```python
from build123d import *
from OCP.BRepFilletAPI import BRepFilletAPI_MakeChamfer

# Parameters (mm, degrees)
SKETCH1_W                   = 2.54
SKETCH1_H                   = 2.5
BOSS_EXTRUDE1_DEPTH         = 8.5
SKETCH2_W                   = 2.54
SKETCH2_H                   = 1.2
CUT_EXTRUDE1_DEPTH          = 0.3
CUT_EXTRUDE2_START          = -6
SKETCH3_W                   = 0.64
SKETCH3_H                   = 0.64
CUT_EXTRUDE2_DEPTH          = 15.68477979
CHAMFER1_SIZE               = 0.5
SKETCH4_W                   = 0.64
SKETCH4_H                   = 0.4
BOSS_EXTRUDE2_DEPTH         = 3.8
CHAMFER2_SIZE               = 1
CHAMFER2_SIZE2              = 0.15838444
LPATTERN1_COUNT             = 9
LPATTERN1_PITCH             = 2.54
CHAMFER1_OF_LPATTERN1_SIZE  = 0.5
CHAMFER2_OF_LPATTERN1_SIZE  = 1
CHAMFER2_OF_LPATTERN1_SIZE2 = 0.15838444


with BuildPart() as part:
    # Sketch1 → Boss-Extrude1 (new body)
    with BuildSketch(Plane(origin=(0, 0, 0), x_dir=(1, 0, 0), z_dir=(0, 1, 0))):
        Rectangle(SKETCH1_W, SKETCH1_H)
    boss_extrude1 = extrude(amount=BOSS_EXTRUDE1_DEPTH)

    # Sketch2 → Cut-Extrude1 (cut)
    with BuildSketch(Plane.XZ):
        Rectangle(SKETCH2_W, SKETCH2_H)
    cut_extrude1 = extrude(amount=-CUT_EXTRUDE1_DEPTH, mode=Mode.SUBTRACT)

    # Sketch3 → Cut-Extrude2 (cut)
    with BuildSketch(Plane(origin=(0, 8.5, 0), x_dir=(1, 0, 0), z_dir=(0, 1, 0)).offset(CUT_EXTRUDE2_START)):
        Rectangle(SKETCH3_W, SKETCH3_H)
    cut_extrude2 = extrude(amount=CUT_EXTRUDE2_DEPTH, mode=Mode.SUBTRACT)

    # Chamfer1
    chamfer1_edges = [part.edges().sort_by_distance(p)[0] for p in [
        (0, 8.5, 0.32),
        (-0.32, 8.5, 0),
        (0, 8.5, -0.32),
        (0.32, 8.5, 0),
    ]]
    chamfer(chamfer1_edges, length=CHAMFER1_SIZE)

    # Sketch4 → Boss-Extrude2 (add)
    with BuildSketch(Plane.XZ.offset(-0.3)):
        Rectangle(SKETCH4_W, SKETCH4_H)
    boss_extrude2 = extrude(amount=BOSS_EXTRUDE2_DEPTH)

    # Chamfer2: one chamfer whose edges measure the first distance from different faces: ONE call of the kernel's chamfer builder (chamfer() names one face for all edges)
    chamfer2_edges_1 = [part.edges().sort_by_distance(p)[0] for p in [
        (0.32, -3.5, 0),
    ]]
    chamfer2_side_1 = [part.faces().sort_by_distance(p)[0] for p in [
        (0.32, -1.6, 0),
    ]]
    chamfer2_edges_2 = [part.edges().sort_by_distance(p)[0] for p in [
        (-0.32, -3.5, 0),
    ]]
    chamfer2_side_2 = [part.faces().sort_by_distance(p)[0] for p in [
        (-0.32, -1.6, 0),
    ]]
    chamfer2 = BRepFilletAPI_MakeChamfer(part.part.solid().wrapped)
    for e in chamfer2_edges_1:
        chamfer2.Add(CHAMFER2_SIZE, CHAMFER2_SIZE2, e.wrapped, chamfer2_side_1[0].wrapped)  # the first distance lies on this face
    for e in chamfer2_edges_2:
        chamfer2.Add(CHAMFER2_SIZE, CHAMFER2_SIZE2, e.wrapped, chamfer2_side_2[0].wrapped)  # the first distance lies on this face
    add(Compound.cast(chamfer2.Shape()), mode=Mode.REPLACE)

    # LPattern1: Boss-Extrude1, Cut-Extrude1, Cut-Extrude2, Boss-Extrude2 ×9
    with Locations(*[(-i * LPATTERN1_PITCH, 0, 0) for i in range(1, LPATTERN1_COUNT)]):
        add(boss_extrude1)
        add(cut_extrude1, mode=Mode.SUBTRACT)
        add(cut_extrude2, mode=Mode.SUBTRACT)
        add(boss_extrude2)

    # Chamfer1 of LPattern1
    chamfer1_of_lpattern1_edges = [part.edges().sort_by_distance(p)[0] for p in [
        (-2.54, 8.5, 0.32),
        (-2.86, 8.5, 0),
        (-2.54, 8.5, -0.32),
        (-2.22, 8.5, 0),
        (-5.08, 8.5, 0.32),
        (-5.4, 8.5, 0),
        (-5.08, 8.5, -0.32),
        (-4.76, 8.5, 0),
        (-7.62, 8.5, 0.32),
        (-7.94, 8.5, 0),
        (-7.62, 8.5, -0.32),
        (-7.3, 8.5, 0),
        (-10.16, 8.5, 0.32),
        (-10.48, 8.5, 0),
        (-10.16, 8.5, -0.32),
        (-9.84, 8.5, 0),
        (-12.7, 8.5, 0.32),
        (-13.02, 8.5, 0),
        (-12.7, 8.5, -0.32),
        (-12.38, 8.5, 0),
        (-15.24, 8.5, 0.32),
        (-15.56, 8.5, 0),
        (-15.24, 8.5, -0.32),
        (-14.92, 8.5, 0),
        (-17.78, 8.5, 0.32),
        (-18.1, 8.5, 0),
        (-17.78, 8.5, -0.32),
        (-17.46, 8.5, 0),
        (-20.32, 8.5, 0.32),
        (-20.64, 8.5, 0),
        (-20.32, 8.5, -0.32),
        (-20, 8.5, 0),
    ]]
    chamfer(chamfer1_of_lpattern1_edges, length=CHAMFER1_OF_LPATTERN1_SIZE)

    # Chamfer2 of LPattern1: one chamfer whose edges measure the first distance from different faces: ONE call of the kernel's chamfer builder (chamfer() names one face for all edges)
    chamfer2_of_lpattern1_edges_1 = [part.edges().sort_by_distance(p)[0] for p in [
        (-2.22, -3.5, 0),
    ]]
    chamfer2_of_lpattern1_side_1 = [part.faces().sort_by_distance(p)[0] for p in [
        (-2.22, -1.6, 0),
    ]]
    chamfer2_of_lpattern1_edges_2 = [part.edges().sort_by_distance(p)[0] for p in [
        (-2.86, -3.5, 0),
    ]]
    chamfer2_of_lpattern1_side_2 = [part.faces().sort_by_distance(p)[0] for p in [
        (-2.86, -1.6, 0),
    ]]
    chamfer2_of_lpattern1_edges_3 = [part.edges().sort_by_distance(p)[0] for p in [
        (-4.76, -3.5, 0),
    ]]
    chamfer2_of_lpattern1_side_3 = [part.faces().sort_by_distance(p)[0] for p in [
        (-4.76, -1.6, 0),
    ]]
    chamfer2_of_lpattern1_edges_4 = [part.edges().sort_by_distance(p)[0] for p in [
        (-5.4, -3.5, 0),
    ]]
    chamfer2_of_lpattern1_side_4 = [part.faces().sort_by_distance(p)[0] for p in [
        (-5.4, -1.6, 0),
    ]]
    chamfer2_of_lpattern1_edges_5 = [part.edges().sort_by_distance(p)[0] for p in [
        (-7.3, -3.5, 0),
    ]]
    chamfer2_of_lpattern1_side_5 = [part.faces().sort_by_distance(p)[0] for p in [
        (-7.3, -1.6, 0),
    ]]
    chamfer2_of_lpattern1_edges_6 = [part.edges().sort_by_distance(p)[0] for p in [
        (-7.94, -3.5, 0),
    ]]
    chamfer2_of_lpattern1_side_6 = [part.faces().sort_by_distance(p)[0] for p in [
        (-7.94, -1.6, 0),
    ]]
    chamfer2_of_lpattern1_edges_7 = [part.edges().sort_by_distance(p)[0] for p in [
        (-9.84, -3.5, 0),
    ]]
    chamfer2_of_lpattern1_side_7 = [part.faces().sort_by_distance(p)[0] for p in [
        (-9.84, -1.6, 0),
    ]]
    chamfer2_of_lpattern1_edges_8 = [part.edges().sort_by_distance(p)[0] for p in [
        (-10.48, -3.5, 0),
    ]]
    chamfer2_of_lpattern1_side_8 = [part.faces().sort_by_distance(p)[0] for p in [
        (-10.48, -1.6, 0),
    ]]
    chamfer2_of_lpattern1_edges_9 = [part.edges().sort_by_distance(p)[0] for p in [
        (-12.38, -3.5, 0),
    ]]
    chamfer2_of_lpattern1_side_9 = [part.faces().sort_by_distance(p)[0] for p in [
        (-12.38, -1.6, 0),
    ]]
    chamfer2_of_lpattern1_edges_10 = [part.edges().sort_by_distance(p)[0] for p in [
        (-13.02, -3.5, 0),
    ]]
    chamfer2_of_lpattern1_side_10 = [part.faces().sort_by_distance(p)[0] for p in [
        (-13.02, -1.6, 0),
    ]]
    chamfer2_of_lpattern1_edges_11 = [part.edges().sort_by_distance(p)[0] for p in [
        (-14.92, -3.5, 0),
    ]]
    chamfer2_of_lpattern1_side_11 = [part.faces().sort_by_distance(p)[0] for p in [
        (-14.92, -1.6, 0),
    ]]
    chamfer2_of_lpattern1_edges_12 = [part.edges().sort_by_distance(p)[0] for p in [
        (-15.56, -3.5, 0),
    ]]
    chamfer2_of_lpattern1_side_12 = [part.faces().sort_by_distance(p)[0] for p in [
        (-15.56, -1.6, 0),
    ]]
    chamfer2_of_lpattern1_edges_13 = [part.edges().sort_by_distance(p)[0] for p in [
        (-17.46, -3.5, 0),
    ]]
    chamfer2_of_lpattern1_side_13 = [part.faces().sort_by_distance(p)[0] for p in [
        (-17.46, -1.6, 0),
    ]]
    chamfer2_of_lpattern1_edges_14 = [part.edges().sort_by_distance(p)[0] for p in [
        (-18.1, -3.5, 0),
    ]]
    chamfer2_of_lpattern1_side_14 = [part.faces().sort_by_distance(p)[0] for p in [
        (-18.1, -1.6, 0),
    ]]
    chamfer2_of_lpattern1_edges_15 = [part.edges().sort_by_distance(p)[0] for p in [
        (-20, -3.5, 0),
    ]]
    chamfer2_of_lpattern1_side_15 = [part.faces().sort_by_distance(p)[0] for p in [
        (-20, -1.6, 0),
    ]]
    chamfer2_of_lpattern1_edges_16 = [part.edges().sort_by_distance(p)[0] for p in [
        (-20.64, -3.5, 0),
    ]]
    chamfer2_of_lpattern1_side_16 = [part.faces().sort_by_distance(p)[0] for p in [
        (-20.64, -1.6, 0),
    ]]
    chamfer2_of_lpattern1 = BRepFilletAPI_MakeChamfer(part.part.solid().wrapped)
    for e in chamfer2_of_lpattern1_edges_1:
        chamfer2_of_lpattern1.Add(CHAMFER2_OF_LPATTERN1_SIZE, CHAMFER2_OF_LPATTERN1_SIZE2, e.wrapped, chamfer2_of_lpattern1_side_1[0].wrapped)  # the first distance lies on this face
    for e in chamfer2_of_lpattern1_edges_2:
        chamfer2_of_lpattern1.Add(CHAMFER2_OF_LPATTERN1_SIZE, CHAMFER2_OF_LPATTERN1_SIZE2, e.wrapped, chamfer2_of_lpattern1_side_2[0].wrapped)  # the first distance lies on this face
    for e in chamfer2_of_lpattern1_edges_3:
        chamfer2_of_lpattern1.Add(CHAMFER2_OF_LPATTERN1_SIZE, CHAMFER2_OF_LPATTERN1_SIZE2, e.wrapped, chamfer2_of_lpattern1_side_3[0].wrapped)  # the first distance lies on this face
    for e in chamfer2_of_lpattern1_edges_4:
        chamfer2_of_lpattern1.Add(CHAMFER2_OF_LPATTERN1_SIZE, CHAMFER2_OF_LPATTERN1_SIZE2, e.wrapped, chamfer2_of_lpattern1_side_4[0].wrapped)  # the first distance lies on this face
    for e in chamfer2_of_lpattern1_edges_5:
        chamfer2_of_lpattern1.Add(CHAMFER2_OF_LPATTERN1_SIZE, CHAMFER2_OF_LPATTERN1_SIZE2, e.wrapped, chamfer2_of_lpattern1_side_5[0].wrapped)  # the first distance lies on this face
    for e in chamfer2_of_lpattern1_edges_6:
        chamfer2_of_lpattern1.Add(CHAMFER2_OF_LPATTERN1_SIZE, CHAMFER2_OF_LPATTERN1_SIZE2, e.wrapped, chamfer2_of_lpattern1_side_6[0].wrapped)  # the first distance lies on this face
    for e in chamfer2_of_lpattern1_edges_7:
        chamfer2_of_lpattern1.Add(CHAMFER2_OF_LPATTERN1_SIZE, CHAMFER2_OF_LPATTERN1_SIZE2, e.wrapped, chamfer2_of_lpattern1_side_7[0].wrapped)  # the first distance lies on this face
    for e in chamfer2_of_lpattern1_edges_8:
        chamfer2_of_lpattern1.Add(CHAMFER2_OF_LPATTERN1_SIZE, CHAMFER2_OF_LPATTERN1_SIZE2, e.wrapped, chamfer2_of_lpattern1_side_8[0].wrapped)  # the first distance lies on this face
    for e in chamfer2_of_lpattern1_edges_9:
        chamfer2_of_lpattern1.Add(CHAMFER2_OF_LPATTERN1_SIZE, CHAMFER2_OF_LPATTERN1_SIZE2, e.wrapped, chamfer2_of_lpattern1_side_9[0].wrapped)  # the first distance lies on this face
    for e in chamfer2_of_lpattern1_edges_10:
        chamfer2_of_lpattern1.Add(CHAMFER2_OF_LPATTERN1_SIZE, CHAMFER2_OF_LPATTERN1_SIZE2, e.wrapped, chamfer2_of_lpattern1_side_10[0].wrapped)  # the first distance lies on this face
    for e in chamfer2_of_lpattern1_edges_11:
        chamfer2_of_lpattern1.Add(CHAMFER2_OF_LPATTERN1_SIZE, CHAMFER2_OF_LPATTERN1_SIZE2, e.wrapped, chamfer2_of_lpattern1_side_11[0].wrapped)  # the first distance lies on this face
    for e in chamfer2_of_lpattern1_edges_12:
        chamfer2_of_lpattern1.Add(CHAMFER2_OF_LPATTERN1_SIZE, CHAMFER2_OF_LPATTERN1_SIZE2, e.wrapped, chamfer2_of_lpattern1_side_12[0].wrapped)  # the first distance lies on this face
    for e in chamfer2_of_lpattern1_edges_13:
        chamfer2_of_lpattern1.Add(CHAMFER2_OF_LPATTERN1_SIZE, CHAMFER2_OF_LPATTERN1_SIZE2, e.wrapped, chamfer2_of_lpattern1_side_13[0].wrapped)  # the first distance lies on this face
    for e in chamfer2_of_lpattern1_edges_14:
        chamfer2_of_lpattern1.Add(CHAMFER2_OF_LPATTERN1_SIZE, CHAMFER2_OF_LPATTERN1_SIZE2, e.wrapped, chamfer2_of_lpattern1_side_14[0].wrapped)  # the first distance lies on this face
    for e in chamfer2_of_lpattern1_edges_15:
        chamfer2_of_lpattern1.Add(CHAMFER2_OF_LPATTERN1_SIZE, CHAMFER2_OF_LPATTERN1_SIZE2, e.wrapped, chamfer2_of_lpattern1_side_15[0].wrapped)  # the first distance lies on this face
    for e in chamfer2_of_lpattern1_edges_16:
        chamfer2_of_lpattern1.Add(CHAMFER2_OF_LPATTERN1_SIZE, CHAMFER2_OF_LPATTERN1_SIZE2, e.wrapped, chamfer2_of_lpattern1_side_16[0].wrapped)  # the first distance lies on this face
    add(Compound.cast(chamfer2_of_lpattern1.Shape()), mode=Mode.REPLACE)


solid = part.part
```
Verification items for the finished model (mm, model axes). Coordinates: 2 decimals unless noted, no trailing zeros. Loops run counter-clockwise (first coordinate to the right, second up) from the corner with the lowest first, then second, coordinate; pieces in that order, holes last. Notation, with made-up numbers: (-24, 65.25) - (16, 65.25) arc R15 cw to (16, 76.25) - close; hole circle Ø1 at (31.5, 87). An arc over 180 degrees is marked (long way). Return JSON: item names as keys, results as strings.
1. Section check B-B, the plane y = 4. Count the separate pieces of the cut face and the enclosed holes in it, then the cut area to 3 significant figures.
Established:
{"separate pieces": "1", "enclosed holes": "9", "area": "53.5 mm2"}
2. Section check A-A, the plane x = -16.5. Record the boundary of the cut face in (y, z), then the cut area to 3 significant figures.
Established:
{"outline": "(0, -1.25) - (8.5, -1.25) - (8.5, 1.25) - (0, 1.25) - (0, 0.6) - (0.3, 0.6) - (0.3, -0.6) - (0, -0.6) - close", "area": "20.9 mm2"}
3. Go/stop test with flat-tipped pins: pin 1 (0.5 mm diameter, centred on x = -5, y = -2, fed in from -Z); pin 2 (0.7 mm diameter, centred on x = -2.5, y = -2, fed in from +Z); pin 3 (5 mm diameter, centred on x = -9, y = -2, fed in from -Z). Record where each tip stops, or that it passes through.
Established:
{"pin 1": "stops at z = -0.2", "pin 2": "stops at z = 0.2", "pin 3": "stops at z = -1.25"}
4. Thickness scan on L1, parallel to Z at x = 0, y = 3.5; L2, parallel to Y at x = -19.25, z = 0.4; L3, parallel to Y at x = -18.25, z = -0.95. Record the ranges inside material, lowest first.
Established:
{"L1": "z = -1.25 to -0.32, 0.32 to 1.25", "L2": "y = 0.3 to 8.5", "L3": "y = 0 to 8.5"}
